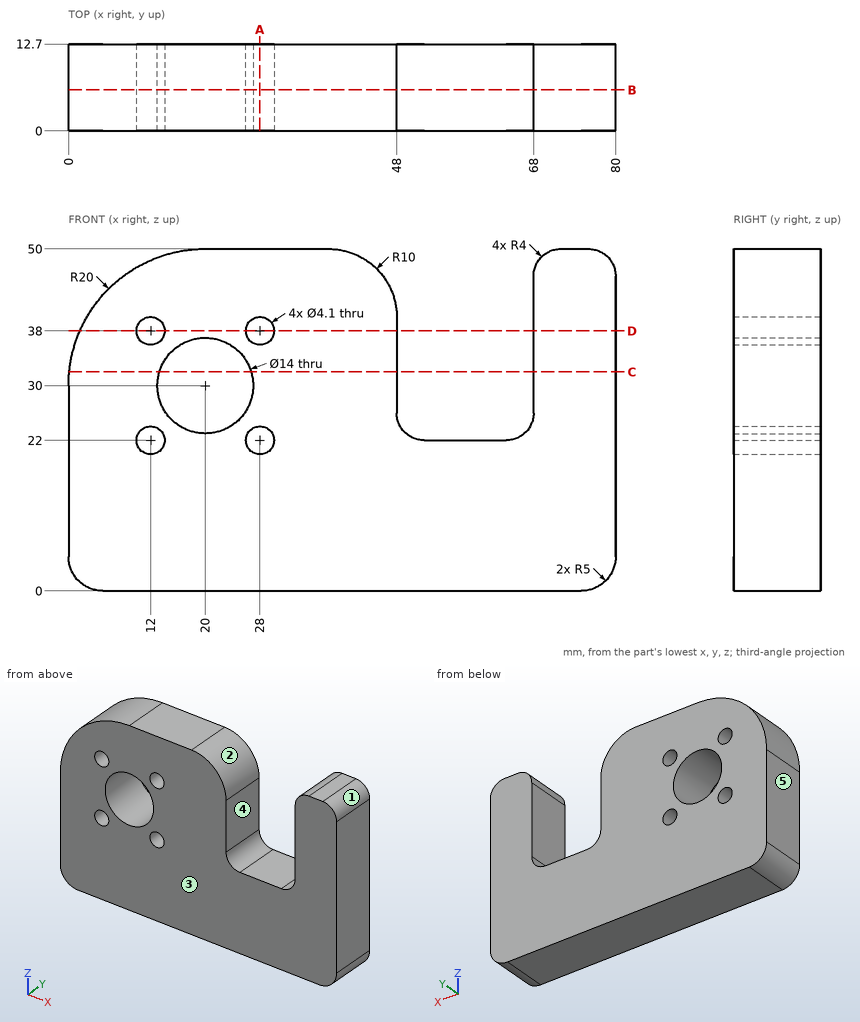
Here's the drawing with two shaded views (mm, measured from the low corner). I have some questions. A direction names the side the tool comes from. Round coordinates to 2 decimals unless told otherwise and drop trailing zeros. Loops run counter-clockwise (first coordinate to the right, second up) from the corner with the lowest first, then second, coordinate; pieces in that order, holes last. Notation, with made-up numbers: (24.25, -30.5) - (62.25, -30.5) arc R12 cw to (62.25, -12.5) - close; hole circle Ø2 at (70.25, 80). An arc over 180 degrees is marked (long way). Use CSV: the item, a comma, the result in double quotes.
Item 1: If we mould it in two halves opening along X, with no side actions, what happens to the marked faces 3, 4 and 5? For each: pulls with the +X half, pulls with the -X half, needs draft (parallel to the pull), parting line crosses it, or undercut.
Here are the results:
face 3,"needs draft"
face 4,"undercut"
face 5,"pulls with the -X half"
Item 2: If we section it at D-D on z = 38: List the corners of the cut face in (x, y) for me, then the cut area to 3 significant figures.
Here are the results:
outline,"(1.67, 0) - (9.95, 0) - (9.95, 12.7) - (1.67, 12.7) - close; (14.05, 0) - (25.95, 0) - (25.95, 12.7) - (14.05, 12.7) - close; (30.05, 0) - (48, 0) - (48, 12.7) - (30.05, 12.7) - close; (68, 0) - (80, 0) - (80, 12.7) - (68, 12.7) - close"
area,"637 mm²"
Item 3: If we section it at B-B on y = 6: List the corners of the cut face in (x, z) for me.
Here are the results:
outline,"(0, 5) arc R5 ccw to (5, 0) - (75, 0) arc R5 ccw to (80, 5) - (80, 46) arc R4 ccw to (76, 50) - (72, 50) arc R4 ccw to (68, 46) - (68, 26) arc R4 cw to (64, 22) - (52, 22) arc R4 cw to (48, 26) - (48, 40) arc R10 ccw to (38, 50) - (20, 50) arc R20 ccw to (0, 30) - close; hole circle Ø4.1 at (12, 22); hole circle Ø4.1 at (12, 38); hole circle Ø14 at (20, 30); hole circle Ø4.1 at (28, 22); hole circle Ø4.1 at (28, 38)"
Item 4: If we section it at A-A on x = 28: List the corners of the cut face in (y, z) for me, then the cut area to 3 significant figures.
Here are the results:
outline,"(0, 0) - (12.7, 0) - (12.7, 19.95) - (0, 19.95) - close; (0, 24.05) - (12.7, 24.05) - (12.7, 35.95) - (0, 35.95) - close; (0, 40.05) - (12.7, 40.05) - (12.7, 50) - (0, 50) - close"
area,"531 mm²"
Item 5: If we section it at C-C on z = 32: List the corners of the cut face in (x, y) for me.
Here are the results:
outline,"(0.1, 0) - (13.29, 0) - (13.29, 12.7) - (0.1, 12.7) - close; (26.71, 0) - (48, 0) - (48, 12.7) - (26.71, 12.7) - close; (68, 0) - (80, 0) - (80, 12.7) - (68, 12.7) - close"
Item 6: For the marked faces 1 and 2, which set-ups out of +Z, -Z, +X, -X, +Y, -Y let a thin tool reach every point of the face, with its end or its side?
Here are the results:
face 1,"+Z, +X, +Y, -Y"
face 2,"+Z, +Y, -Y"
Item 7: I need wall thicknesses on L1, parallel to Z at x = 28, y = 9.25; L2, parallel to X at y = 2.25, z = 34; L3, parallel to Z at x = 12, y = 7. Which ranges of each line are inside material? Lowest first, please. Write a range as [from, to].
Here are the results:
L1,"z = [0, 19.95], [24.05, 35.95], [40.05, 50]"
L2,"x = [0.4, 14.26], [25.74, 48], [68, 80]"
L3,"z = [0, 19.95], [24.05, 35.95], [40.05, 48.33]"
Item 8: Will this pin go through, and if not, where does the flat tip stop? pin 1 (6.5 mm diameter, centred on y = 6, z = 33.5, fed in from -X).
Here are the results:
pin 1,"stops at x = 0"
